The listing builds one solid part. Answer for the finished solid, in the listing's coordinates (mm). A direction names the side the tool comes from. Coordinates: 2 decimals unless noted, no trailing zeros. Order: outer loops, then holes, each group sorted by start corner. A loop starts at its lowest first (then second) coordinate and runs counter-clockwise, first axis right, second up.
from build123d import *

# Parameters (mm, degrees)
F1_DEPTH  = 50.8
F2_R      = 6.35
F3_DEPTH  = 50.8
F5_DEPTH  = 152.4
F7_DEPTH  = 152.4
F9_DEPTH  = 25.4
F11_DEPTH = 25.4
F13_DEPTH = 25.4


with BuildPart() as f1:
    # F0 (on Front) → F1 (new body, symmetric)
    with BuildSketch(Plane.XZ):
        Polygon((-76.2, 50.8), (-76.2, 0), (-38.1, 0), (-38.1, 12.7), (0, 12.7), (38.1, 12.7), (38.1, 0), (76.2, 0), (76.2, 50.8), align=None)
    extrude(amount=F1_DEPTH, both=True)

    # F2 (on face) → F3 (cut)
    with BuildSketch(Plane.XY.offset(50.8)):
        with Locations((-57.15, -31.75)):
            Circle(F2_R)
        with Locations((57.15, -31.75)):
            Circle(F2_R)
    extrude(amount=-F3_DEPTH, mode=Mode.SUBTRACT)

    # F4 (on face) → F5 (cut)
    with BuildSketch(Plane.YZ.offset(76.2)):
        Polygon((-12.7, 38.1), (-12.7, 25.4), (38.1, 25.4), (38.1, 38.1), (22.225, 38.1), (22.225, 50.8), (3.175, 50.8), (3.175, 38.1), align=None)
    extrude(amount=-F5_DEPTH, mode=Mode.SUBTRACT)

    # F6 (on face) → F7 (join)
    with BuildSketch(Plane.YZ.offset(76.2)):
        Polygon((50.8, 101.6), (50.8, 50.8), (50.8, 0), (76.2, 0), (76.2, 101.6), align=None)
    extrude(amount=-F7_DEPTH)

    # F8 (on face) → F9 (cut)
    with BuildSketch(Plane(origin=(0, 76.2, 0), x_dir=(-1, 0, 0), z_dir=(0, 1, 0))):
        with BuildLine():
            Line((38.1, 101.6), (-38.1, 101.6))
            ThreePointArc((-38.1, 101.6), (0, 63.5), (38.1, 101.6))
        make_face()
    extrude(amount=-F9_DEPTH, mode=Mode.SUBTRACT)

    # F10 (on face) → F11 (cut)
    with BuildSketch(Plane(origin=(0, 76.2, 0), x_dir=(-1, 0, 0), z_dir=(0, 1, 0))):
        with BuildLine():
            ThreePointArc((63.5, 101.6), (72.480256, 97.880256), (76.2, 88.9))
            Line((76.2, 88.9), (76.2, 101.6))
            Line((76.2, 101.6), (63.5, 101.6))
        make_face()
    extrude(amount=-F11_DEPTH, mode=Mode.SUBTRACT)

    # F12 (on face) → F13 (cut)
    with BuildSketch(Plane(origin=(0, 76.2, 0), x_dir=(-1, 0, 0), z_dir=(0, 1, 0))):
        with BuildLine():
            ThreePointArc((-76.2, 88.9), (-72.480256, 97.880256), (-63.5, 101.6))
            Line((-63.5, 101.6), (-76.2, 101.6))
            Line((-76.2, 101.6), (-76.2, 88.9))
        make_face()
    extrude(amount=-F13_DEPTH, mode=Mode.SUBTRACT)


solid = f1.part
1) Section D-D (z = 91.5) is taken. Give the vertices of the cut face in (x, y), then the cut area to 3 significant figures.
2) Each of these flat-tipped pins is pushed along its axis until it touches: P1, Ø2, axis at x = 8, y = -17, coming from the -Z side; P2, Ø7.5, axis at x = 57.15, y = -31.75, coming from the +Z side; P3, Ø8.5, axis at x = -33, y = 31.5, coming from the +Z side; P4, Ø6, axis at x = -53, z = 63.5, coming from the -Y side. Where does it stop, or does it pass through?
3) A tool of negligible diameter and unlimited length cuts with its end or side. For faces 1 (the face through (1, 50.8, 6)), 2 (the face through (1, 36, 50.8)), 3 (the face through (1, 22.225, 44)), 4 (the face through (1, -12.7, 32)), from which of +Z, -Z, +X, -X, +Y, -Y can it reach the whole face along a straight path? Write none if from no direction.
4) Section A-A (x = 57.15) is taken. Give the vertices of the cut face in (y, z) (3 decimals).
5) Consider L1, parallel to X at y = -31, z = 27; L2, parallel to Y at x = 57, z = 31; L3, parallel to Z at x = 17, y = -6. Determine where each line is inside the solid, lowest interval first.
6) Determine the mould class of faces 5 (the face through (0.84, 63.68, 63.51)), 6 (the face through (1, 76.2, 39)), 7 (the face through (1, -5, 38.1)), 8 (the face through (1, 38.1, 32)) for opening direction Z: released by +Z, released by -Z, zero draft, split by the parting line, or undercut.
7) Section B-B (y = -31.75) is taken. Give the vertices of the cut face in (x, z).
8) Section C-C (x = 0) is taken. Give the vertices of the cut face in (y, z) (3 decimals), then the cut area to 3 significant figures.
Filled sheet:
1. outline: (-75.93, 50.8) - (-36.74, 50.8) - (-36.74, 76.2) - (-75.93, 76.2) - close; (36.74, 50.8) - (75.93, 50.8) - (75.93, 76.2) - (36.74, 76.2) - close
1. area: 1,990 mm2
2. P1: stops at z = 12.7
2. P2: passes through
2. P3: stops at z = 50.8
2. P4: stops at y = 50.8
3. face 1: -Z, -Y
3. face 2: +Z, +X, -X, -Y
3. face 3: +Z, +X, -X
3. face 4: +X, -X
4. outline: (-50.8, 0) - (-38.1, 0) - (-38.1, 50.8) - (-50.8, 50.8) - close; (-25.4, 0) - (76.2, 0) - (76.2, 101.6) - (50.8, 101.6) - (50.8, 50.8) - (22.225, 50.8) - (22.225, 38.1) - (38.1, 38.1) - (38.1, 25.4) - (-12.7, 25.4) - (-12.7, 38.1) - (3.175, 38.1) - (3.175, 50.8) - (-25.4, 50.8) - close
5. L1: x = -76.2 to -63.46, -50.84 to 50.84, 63.46 to 76.2
5. L2: y = -50.8 to -38.1, -25.4 to -12.7, 38.1 to 76.2
5. L3: z = 12.7 to 25.4, 38.1 to 50.8
6. face 5: released by +Z
6. face 6: zero draft
6. face 7: undercut
6. face 8: undercut
7. outline: (-76.2, 0) - (-63.5, 0) - (-63.5, 50.8) - (-76.2, 50.8) - close; (-50.8, 0) - (-38.1, 0) - (-38.1, 12.7) - (38.1, 12.7) - (38.1, 0) - (50.8, 0) - (50.8, 50.8) - (-50.8, 50.8) - close; (63.5, 0) - (76.2, 0) - (76.2, 50.8) - (63.5, 50.8) - close
8. outline: (-50.8, 12.7) - (50.8, 12.7) - (50.8, 0) - (76.2, 0) - (76.2, 63.5) - (50.8, 63.5) - (50.8, 50.8) - (22.225, 50.8) - (22.225, 38.1) - (38.1, 38.1) - (38.1, 25.4) - (-12.7, 25.4) - (-12.7, 38.1) - (3.175, 38.1) - (3.175, 50.8) - (-50.8, 50.8) - close
8. area: 4,600 mm2
